Check sheet for the modelled part. Datum: model origin and axes. Units: mm. Coordinates: 2 decimals unless noted, no trailing zeros. Loops run counter-clockwise (first coordinate to the right, second up) from the corner with the lowest first, then second, coordinate; pieces in that order, holes last. Notation, with made-up numbers: (-1.75, 48) -> (29.25, 48) arc R27 ccw to (29.25, 81) -> close; hole circle Ø11 at (41, 49). An arc over 180 degrees is marked (long way). Use CSV: the item, a comma, the result in double quotes.
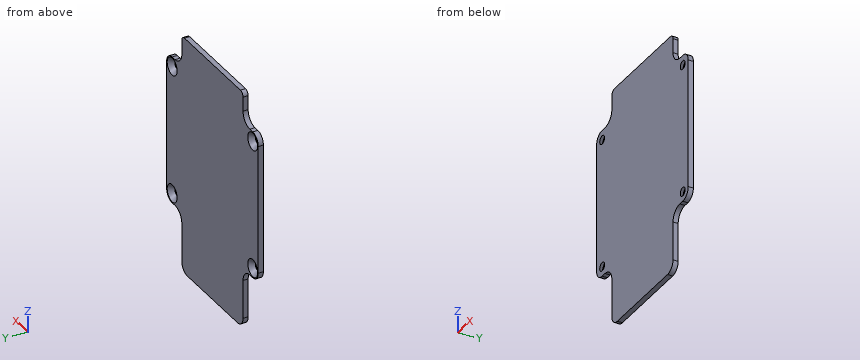
```python
from build123d import *

# Parameters (mm, degrees)
BOSS_EXTRUDE3_DEPTH                            = 1.6
CSK_FOR_2_FLAT_HEAD_MACHINE_SCREW1_D           = 2.4384
CSK_FOR_2_FLAT_HEAD_MACHINE_SCREW1_DEPTH       = 5.588
CSK_FOR_2_FLAT_HEAD_MACHINE_SCREW1_CSINK_D     = 5.461
CSK_FOR_2_FLAT_HEAD_MACHINE_SCREW1_CSINK_ANGLE = 82
CSK_FOR_2_FLAT_HEAD_MACHINE_SCREW1_TIP         = 0.732569267


with BuildPart() as part:
    # Sketch1 → Boss-Extrude3 (new body)
    with BuildSketch(Plane(origin=(0, 9.525, 0), x_dir=(1, 0, 0), z_dir=(0, 1, 0))):
        with BuildLine():
            Line((-16.891, 39.0525), (-16.891, 26.9875))
            ThreePointArc((-16.891, 26.9875), (-17.988324444, 24.338324444), (-20.6375, 23.241))
            Line((-20.6375, 23.241), (-22.225, 23.241))
            ThreePointArc((-22.225, 23.241), (-24.380261469, 22.348261469), (-25.273, 20.193))
            Line((-25.273, 20.193), (-25.273, -20.193))
            ThreePointArc((-25.273, -20.193), (-24.380261469, -22.348261469), (-22.225, -23.241))
            Line((-22.225, -23.241), (-20.6375, -23.241))
            ThreePointArc((-20.6375, -23.241), (-17.988324444, -24.338324444), (-16.891, -26.9875))
            Line((-16.891, -26.9875), (-16.891, -31.4325))
            ThreePointArc((-16.891, -31.4325), (-16.463229454, -32.465229454), (-15.4305, -32.893))
            Line((-15.4305, -32.893), (15.4305, -32.893))
            ThreePointArc((15.4305, -32.893), (16.463229454, -32.465229454), (16.891, -31.4325))
            Line((16.891, -31.4325), (16.891, -26.9875))
            ThreePointArc((16.891, -26.9875), (17.988324444, -24.338324444), (20.6375, -23.241))
            Line((20.6375, -23.241), (22.225, -23.241))
            ThreePointArc((22.225, -23.241), (24.380261469, -22.348261469), (25.273, -20.193))
            Line((25.273, -20.193), (25.273, 20.193))
            ThreePointArc((25.273, 20.193), (24.380261469, 22.348261469), (22.225, 23.241))
            Line((22.225, 23.241), (20.6375, 23.241))
            ThreePointArc((20.6375, 23.241), (17.988324444, 24.338324444), (16.891, 26.9875))
            Line((16.891, 26.9875), (16.891, 39.0525))
            ThreePointArc((16.891, 39.0525), (15.998261469, 41.207761469), (13.843, 42.1005))
            Line((13.843, 42.1005), (-13.843, 42.1005))
            ThreePointArc((-13.843, 42.1005), (-15.998261469, 41.207761469), (-16.891, 39.0525))
        make_face()
    extrude(amount=-BOSS_EXTRUDE3_DEPTH)

    # CSK for #2 Flat Head Machine Screw1
    with Locations(Plane(origin=(22.225, 9.525, 20.193), x_dir=(0, 0, 1), z_dir=(0, 1, 0))):
        with Locations((0, 0), (0, -44.45), (-40.386, -44.45), (-40.386, 0)):
            CounterSinkHole(CSK_FOR_2_FLAT_HEAD_MACHINE_SCREW1_D / 2, CSK_FOR_2_FLAT_HEAD_MACHINE_SCREW1_CSINK_D / 2, depth=CSK_FOR_2_FLAT_HEAD_MACHINE_SCREW1_DEPTH, counter_sink_angle=CSK_FOR_2_FLAT_HEAD_MACHINE_SCREW1_CSINK_ANGLE)
            with Locations((0, 0, -(CSK_FOR_2_FLAT_HEAD_MACHINE_SCREW1_DEPTH + CSK_FOR_2_FLAT_HEAD_MACHINE_SCREW1_TIP / 2))):  # 118° drill point
                Cone(0, CSK_FOR_2_FLAT_HEAD_MACHINE_SCREW1_D / 2, CSK_FOR_2_FLAT_HEAD_MACHINE_SCREW1_TIP, mode=Mode.SUBTRACT)


solid = part.part
```
1) Cross-section at C-C on x = -18.5. Record the boundary of the cut face in (y, z) (3 decimals), and give its area (3 significant figures).
Answer below:
outline,"(7.925, -23.911) -> (9.525, -23.911) -> (9.525, 23.911) -> (7.925, 23.911) -> close"
area,"76.5 mm²"
2) Cross-section at B-B on z = -28. Record the boundary of the cut face in (x, y) (3 decimals), and give its area (3 significant figures).
Answer below:
outline,"(-16.891, 7.925) -> (16.891, 7.925) -> (16.891, 9.525) -> (-16.891, 9.525) -> close"
area,"54.1 mm²"
3) Cross-section at A-A on y = 8.2. Record the boundary of the cut face in (x, z) (1 decimal), and give its area (3 significant figures).
Answer below:
outline,"(-25.3, -20.2) arc R3 ccw to (-22.2, -23.2) -> (-20.6, -23.2) arc R3.7 cw to (-16.9, -27) -> (-16.9, -39.1) arc R3 ccw to (-13.8, -42.1) -> (13.8, -42.1) arc R3 ccw to (16.9, -39.1) -> (16.9, -27) arc R3.7 cw to (20.6, -23.2) -> (22.2, -23.2) arc R3 ccw to (25.3, -20.2) -> (25.3, 20.2) arc R3 ccw to (22.2, 23.2) -> (20.6, 23.2) arc R3.7 cw to (16.9, 27) -> (16.9, 31.4) arc R1.5 ccw to (15.4, 32.9) -> (-15.4, 32.9) arc R1.5 ccw to (-16.9, 31.4) -> (-16.9, 27) arc R3.7 cw to (-20.6, 23.2) -> (-22.2, 23.2) arc R3 ccw to (-25.3, 20.2) -> close; hole circle Ø3.2 at (-22.2, -20.2); hole circle Ø3.2 at (-22.2, 20.2); hole circle Ø3.2 at (22.2, -20.2); hole circle Ø3.2 at (22.2, 20.2)"
area,"3,280 mm²"
4) Thickness scan on line 1 along Z through (x, y) = (22, 9.15); line 2 along X through (y, z) = (8.5, 28); line 3 along X through (y, z) = (8.4, 25). Record the ranges inside material, lowest first. Write a range as from..to.
Answer below:
line 1,"z = -23.24..-22.59, -17.8..17.8, 22.59..23.24"
line 2,"x = -16.89..16.89"
line 3,"x = -17.46..17.46"
5) Go/stop test with flat-tipped pins: pin 1 Ø0.5 at (y, z) = (8.5, 29.5) entering from +X; pin 2 Ø0.8 at (y, z) = (8.5, 29.5) entering from -X. Record where each tip stops, or that it passes through.
Answer below:
pin 1,"stops at x = 16.89"
pin 2,"stops at x = -16.89"
